from build123d import *

# Parameters (mm, degrees)
ESQUISSE2_R        = 43.50000000000001
ESQUISSE2_R_2      = 40.5
BOSS_EXTRU_1_DEPTH = 10
BOSS_EXTRU_2_START = -3
ESQUISSE2_2_R      = 43.50000000000001
BOSS_EXTRU_2_DEPTH = 3
BOSS_EXTRU_3_DEPTH = 12
BOSS_EXTRU_4_START = 12
BOSS_EXTRU_4_DEPTH = 7.5
BOSS_EXTRU_5_START = 19.5
BOSS_EXTRU_5_DEPTH = 3
BOSS_EXTRU_6_START = 22.5
BOSS_EXTRU_6_DEPTH = 3


with BuildPart() as part:
    # Esquisse2 → Boss.-Extru.1 (new body)
    with BuildSketch(Plane(origin=(0, 0, 0), x_dir=(0, 0, -1), z_dir=(1, 0, 0))):
        Circle(ESQUISSE2_R)
        Circle(ESQUISSE2_R_2, mode=Mode.SUBTRACT)
    extrude(amount=BOSS_EXTRU_1_DEPTH)

    # Esquisse2<2> → Boss.-Extru.2 (add)
    with BuildSketch(Plane(origin=(0, 0, 0), x_dir=(0, 0, -1), z_dir=(1, 0, 0)).offset(BOSS_EXTRU_2_START)):
        Circle(ESQUISSE2_2_R)
    extrude(amount=BOSS_EXTRU_2_DEPTH)

    # Esquisse3 → Boss.-Extru.3 (add)
    with BuildSketch(Plane(origin=(0, 0, 0), x_dir=(0, 0, -1), z_dir=(1, 0, 0))):
        with BuildLine():
            Line((26.11118120318316, 15.522854869939358), (26.11118120318316, 17.022854869939355))
            ThreePointArc((26.111181203183165, 17.02285486993936), (12.199019622456863, 19.70655185145899), (3.55e-15, 12.500000000000004))
            ThreePointArc((3.55e-15, 12.500000000000002), (-4.387505004004, 4.4e-16), (5.33e-15, -12.5))
            Line((3.55e-15, -12.5), (8.54855768792795, -23.17714513006065))
            Line((8.54855768792795, -23.17714513006065), (13.000000000000005, -23.17714513006065))
            Line((13.000000000000005, -23.177145130060648), (13.000000000000004, -16.97714513006065))
            Line((13.000000000000004, -16.97714513006065), (13.000000000000004, -15.677145130060648))
            ThreePointArc((13.000000000000004, -15.677145130060646), (3.4519983220891106, 6.690070139129679), (26.111181203183158, 15.522854869939358))
        make_face()
    extrude(amount=BOSS_EXTRU_3_DEPTH)

    # Esquisse3<3> → Boss.-Extru.4 (add)
    with BuildSketch(Plane(origin=(0, 0, 0), x_dir=(0, 0, -1), z_dir=(1, 0, 0)).offset(BOSS_EXTRU_4_START)):
        with BuildLine():
            Line((26.11118120318316, 17.022854869939355), (26.11118120318316, 6.022854869939354))
            Line((26.11118120318316, 6.022854869939354), (13, 6.022854869939352))
            Line((13, 6.022854869939352), (13.000000000000004, -16.97714513006065))
            Line((13.000000000000004, -16.97714513006065), (26.111181203183165, -16.97714513006065))
            Line((26.111181203183165, -16.97714513006065), (26.11118120318317, -23.177145130060648))
            Line((26.11118120318317, -23.177145130060648), (8.54855768792795, -23.17714513006065))
            Line((8.54855768792795, -23.17714513006065), (3.37e-15, -12.5))
            ThreePointArc((3.37e-15, -12.5), (-4.387505004004002, -2.45e-15), (3.37e-15, 12.5))
            ThreePointArc((3.37e-15, 12.5), (12.199019622456856, 19.70655185145899), (26.11118120318316, 17.022854869939355))
        make_face()
    extrude(amount=BOSS_EXTRU_4_DEPTH)

    # Esquisse3<4> → Boss.-Extru.5 (add)
    with BuildSketch(Plane(origin=(0, 0, 0), x_dir=(0, 0, -1), z_dir=(1, 0, 0)).offset(BOSS_EXTRU_5_START)):
        with BuildLine():
            Line((26.11118120318316, 11.322854869939354), (26.11118120318316, 15.522854869939358))
            ThreePointArc((26.111181203183158, 15.522854869939358), (3.4519983220891106, 6.690070139129679), (13.000000000000004, -15.677145130060646))
            Line((13.000000000000004, -15.677145130060648), (13, 6.022854869939352))
            Line((13, 6.022854869939352), (13, 11.322854869939354))
            Line((13, 11.322854869939354), (26.11118120318316, 11.322854869939354))
        make_face()
        with BuildLine():
            Line((26.11118120318316, 15.522854869939358), (26.11118120318316, 17.022854869939355))
            ThreePointArc((26.111181203183165, 17.02285486993936), (12.199019622456863, 19.70655185145899), (3.55e-15, 12.500000000000004))
            ThreePointArc((3.55e-15, 12.500000000000002), (-4.387505004004, 4.4e-16), (5.33e-15, -12.5))
            Line((3.55e-15, -12.5), (8.54855768792795, -23.17714513006065))
            Line((8.54855768792795, -23.17714513006065), (13.000000000000005, -23.17714513006065))
            Line((13.000000000000005, -23.177145130060648), (13.000000000000004, -16.97714513006065))
            Line((13.000000000000004, -16.97714513006065), (13.000000000000004, -15.677145130060648))
            ThreePointArc((13.000000000000004, -15.677145130060646), (3.4519983220891106, 6.690070139129679), (26.111181203183158, 15.522854869939358))
        make_face()
    extrude(amount=BOSS_EXTRU_5_DEPTH)

    # Esquisse3<5> → Boss.-Extru.6 (add)
    with BuildSketch(Plane(origin=(0, 0, 0), x_dir=(0, 0, -1), z_dir=(1, 0, 0)).offset(BOSS_EXTRU_6_START)):
        Polygon((26.111181203183165, -16.97714513006065), (13.000000000000004, -16.97714513006065), (13.000000000000005, -23.177145130060648), (26.11118120318317, -23.177145130060648), align=None)
        with BuildLine():
            Line((26.11118120318316, 15.522854869939358), (26.11118120318316, 17.022854869939355))
            ThreePointArc((26.111181203183165, 17.02285486993936), (12.199019622456863, 19.70655185145899), (3.55e-15, 12.500000000000004))
            ThreePointArc((3.55e-15, 12.500000000000002), (-4.387505004004, 4.4e-16), (5.33e-15, -12.5))
            Line((3.55e-15, -12.5), (8.54855768792795, -23.17714513006065))
            Line((8.54855768792795, -23.17714513006065), (13.000000000000005, -23.17714513006065))
            Line((13.000000000000005, -23.177145130060648), (13.000000000000004, -16.97714513006065))
            Line((13.000000000000004, -16.97714513006065), (13.000000000000004, -15.677145130060648))
            ThreePointArc((13.000000000000004, -15.677145130060646), (3.4519983220891106, 6.690070139129679), (26.111181203183158, 15.522854869939358))
        make_face()
        with BuildLine():
            Line((26.11118120318316, 11.322854869939354), (26.11118120318316, 15.522854869939358))
            ThreePointArc((26.111181203183158, 15.522854869939358), (3.4519983220891106, 6.690070139129679), (13.000000000000004, -15.677145130060646))
            Line((13.000000000000004, -15.677145130060648), (13, 6.022854869939352))
            Line((13, 6.022854869939352), (13, 11.322854869939354))
            Line((13, 11.322854869939354), (26.11118120318316, 11.322854869939354))
        make_face()
        Polygon((26.11118120318316, 6.022854869939355), (26.11118120318316, 11.322854869939354), (13, 11.322854869939354), (13, 6.022854869939352), align=None)
    extrude(amount=BOSS_EXTRU_6_DEPTH)


solid = part.part
Read the model definition and answer for the solid it produces. Units are mm, in the model's axes. A direction names the side the tool comes from. Give positions to 0.01 mm unless a question says otherwise; leave off trailing zeros. Write each loop counter-clockwise with the first axis right and the second up, starting at its lowest first coordinate (ties: lowest second). Pieces come first, ordered by that corner, then holes. Notation, with made-up numbers: (-11, 43.5) - (0, 43.5) arc R21 cw to (0, 47.5) - close; hole circle Ø1 at (-38.5, 53). An arc over 180 degrees is marked (long way). Return JSON: item names as keys, results as strings.
Q1. For faces 1 (the face through (3.41, 43.13, 5.66)), 2 (the face through (16, -16.977, -19)), 3 (the face through (-3, 1, 1)), 4 (the face through (22.5, 9, -19)), 5 (the face through (10, -29, -29)), determine the directions among +Z, -Z, +X, -X, +Y, -Y from which every point of the face is accessible in a straight line to the end or side of a thin tool.
Reply:
{"face 1": "+X, -X", "face 2": "-Z, +X", "face 3": "+Z, -Z, -X, +Y, -Y", "face 4": "-Z, -Y", "face 5": "+X"}
Q2. Given P1, Ø3.5, axis at x = 24.5, z = -18, coming from the -Y side; P2, Ø3.5, axis at x = 24.5, y = -20.5, coming from the -Z side; P3, Ø8, axis at y = 29.5, z = 20, coming from the +X side; P4, Ø8, axis at y = -2.5, z = -14.5, coming from the +X side, each flat-ended and moving along its own axis, determine where each tip first touches the part or whether it passes through.
Reply:
{"P1": "y = -23.18", "P2": "z = -26.11", "P3": "x = 0", "P4": "x = 25.5"}
Q3. Consider line 1 along X through (y, z) = (8, -18); line 2 along Y through (x, z) = (2.5, 0); line 3 along Y through (x, z) = (4.75, -3.5) (1 decimal). Determine where each line is inside the solid, lowest interval first. Write a range as [from, to].
Reply:
{"line 1": "[-3, 0], [12, 19.5], [22.5, 25.5]", "line 2": "[-43.5, -40.5], [-12.5, 12.5], [40.5, 43.5]", "line 3": "[-43.4, -40.3], [-16.9, -6.5], [6.8, 15.9], [40.3, 43.4]"}
Q4. A cutting plane is placed at A-A, the plane x = 3.5. Determine the outline of the cut face in (y, z).
Reply:
{"outline": "circle Ø87 at (0, 0); (-23.18, -13) - (-15.68, -13) arc R16.93 cw (long way) to (15.52, -26.11) - (17.02, -26.11) arc R20 ccw to (-12.5, 0) - (-23.18, -8.55) - close; hole circle Ø81 at (0, 0)"}
Q5. A cutting plane is placed at D-D, the plane y = 0. Determine the outline of the cut face in (x, z).
Reply:
{"outline": "(-3, -43.5) - (10, -43.5) - (10, -40.5) - (0, -40.5) - (0, -2.13) - (12, -2.13) - (12, -13) - (25.5, -13) - (25.5, 4.39) - (0, 4.39) - (0, 40.5) - (10, 40.5) - (10, 43.5) - (-3, 43.5) - close"}
Q6. A cutting plane is placed at B-B, the plane z = -19. Determine the outline of the cut face in (x, y), and give its area (3 significant figures).
Reply:
{"outline": "(-3, -39.13) - (10, -39.13) - (10, -35.77) - (0, -35.77) - (0, 17.06) - (12, 17.06) - (12, 6.02) - (19.5, 6.02) - (19.5, 11.32) - (22.5, 11.32) - (22.5, 6.02) - (25.5, 6.02) - (25.5, 19.71) - (0, 19.71) - (0, 35.77) - (10, 35.77) - (10, 39.13) - (-3, 39.13) - close; (12, -23.18) - (19.5, -23.18) - (19.5, -16.98) - (12, -16.98) - close; (22.5, -23.18) - (25.5, -23.18) - (25.5, -16.98) - (22.5, -16.98) - close", "area": "568 mm²"}
Q7. A cutting plane is placed at C-C, the plane x = 15.5. Determine the outline of the cut face in (y, z), and give its area (3 significant figures).
Reply:
{"outline": "(-23.18, -26.11) - (-16.98, -26.11) - (-16.98, -13) - (6.02, -13) - (6.02, -26.11) - (17.02, -26.11) arc R20 ccw to (-12.5, 0) - (-23.18, -8.55) - close", "area": "809 mm²"}
Q8. For a pull along Z with two mould halves and no side action, classify faces 6 (the face through (24, -20, -26.111)), 7 (the face through (0, 1, -8)), 8 (the face through (12.57, -17.76, -4.21)), 9 (the face through (25.5, -1, -11)) as released by +Z, released by -Z, zero draft, split by the parting line, or undercut.
Reply:
{"face 6": "released by -Z", "face 7": "undercut", "face 8": "undercut", "face 9": "zero draft"}
